from build123d import *

# Parameters (mm, degrees)
F1_DEPTH = 100


with BuildPart() as f1:
    # F0 (on Right) → F1 (new body)
    with BuildSketch(Plane.YZ):
        Polygon((2.998335, 3.96), (0, 3.96), (-2.998335, 3.96), (-6, 6.961665), (-6, 8), (-3, 8), (-3, 10), (-10, 10), (-10, 3), (-8, 3), (-8, 6), (-6.961665, 6), (-3.96, 2.998335), (-3.96, 0), (-3.96, -2.998335), (-6.961665, -6), (-8, -6), (-8, -3), (-10, -3), (-10, -10), (-3, -10), (-3, -8), (-6, -8), (-6, -6.961665), (-2.998335, -3.96), (0, -3.96), (2.998335, -3.96), (6, -6.961665), (6, -8), (3, -8), (3, -10), (10, -10), (10, -3), (8, -3), (8, -6), (6.961665, -6), (3.96, -2.998335), (3.96, 0), (3.96, 2.998335), (6.961665, 6), (8, 6), (8, 3), (10, 3), (10, 10), (3, 10), (3, 8), (6, 8), (6, 6.961665), align=None)
    extrude(amount=F1_DEPTH)


solid = f1.part
For this review, take the finished solid that the model builds, in its own axes (mm). A direction names the side the tool comes from. Coordinates: 2 decimals unless noted, no trailing zeros. Loops run counter-clockwise (first coordinate to the right, second up) from the corner with the lowest first, then second, coordinate; pieces in that order, holes last. Notation, with made-up numbers: (66.5, -9) - (123.5, -9) arc R25 ccw to (123.5, 5) - close; hole circle Ø6 at (41, 55.25). An arc over 180 degrees is marked (long way). Use a Markdown table: item, result. Add a question column.
Item 1: Tool access review of faces 4 (the face through (49, -9, -3)), 5 (the face through (49, 7, 10)), 6 (the face through (49, 3, -9)), 7 (the face through (49.3, -5.48, 4.52)): name each direction out of +Z, -Z, +X, -X, +Y, -Y from which nothing blocks a thin tool from reaching the whole face with its end or side.
Item 2: For line 1 (Y direction, x = 35, z = -7); line 2 (Z direction, x = 26, y = 3.5); line 3 (Z direction, x = 39.5, y = -8.75), list the stretches that pass through material, from the lowest coordinate up.
Item 3: We need section A-A (z = 0.75). Give the boundary of the cut face in (x, y), and give its area (3 significant figures).
Item 4: Mouldability with a two-part tool opening along Y and no side actions: class faces 1 (the face through (49, 9, -3)), 2 (the face through (49, 0, 3.96)), 3 (the face through (49, -10, 7)) as pulls with the +Y half, pulls with the -Y half, needs draft (parallel to the pull), parting line crosses it, or undercut.
Results list:
| question | item | result |
|---|---|---|
| 1 | face 4 | +X, -X, -Y |
| 1 | face 5 | +Z, +X, -X, +Y, -Y |
| 1 | face 6 | -Z, +X, -X |
| 1 | face 7 | +X, -X |
| 2 | line 1 | y = -10 to -6, 6 to 10 |
| 2 | line 2 | z = -10 to -8, -4.46 to 4.46, 8 to 10 |
| 2 | line 3 | z = -10 to -3, 3 to 10 |
| 3 | outline | (0, -3.96) - (100, -3.96) - (100, 3.96) - (0, 3.96) - close |
| 3 | area | 792 mm^2 |
| 4 | face 1 | needs draft |
| 4 | face 2 | undercut |
| 4 | face 3 | pulls with the -Y half |
